from build123d import *

# Parameters (mm, degrees)
F0_R     = 9.525
F1_DEPTH = 6.35


with BuildPart() as f1:
    # F0 (on Front) → F1 (new body)
    with BuildSketch(Plane.XZ):
        with BuildLine():
            Line((0.076142, 15.237411), (0.853466, 15.24))
            Line((0.853466, 15.24), (45.610599, 15.24))
            ThreePointArc((45.610599, 15.24), (58.968483, 24.02141), (74.599698, 27.369742))
            ThreePointArc((74.599698, 27.369742), (81.067987, 24.723293), (84.296649, 18.525051))
            Line((84.296649, 18.525051), (140.869953, 18.525051))
            Line((140.869953, 18.525051), (140.869953, 1.794949))
            Line((140.869953, 1.794949), (140.869953, -1.794949))
            Line((140.869953, -1.794949), (140.869953, -18.525051))
            Line((140.869953, -18.525051), (84.296649, -18.525051))
            ThreePointArc((84.296649, -18.525051), (81.067987, -24.723293), (74.599698, -27.369742))
            ThreePointArc((74.599698, -27.369742), (58.968483, -24.02141), (45.610599, -15.24))
            Line((45.610599, -15.24), (0.853466, -15.24))
            Line((0.853466, -15.24), (0.076142, -15.237411))
            Line((0.076142, -15.237411), (0.000423, -37.973113))
            ThreePointArc((0.000423, -37.973113), (0.000106, -38.036556), (0, -38.1))
            ThreePointArc((0, -38.1), (5.576611, -51.567379), (19.041501, -57.149998))
            Line((19.041501, -57.149998), (107.941492, -57.189659))
            Line((107.941492, -57.189659), (148.581492, -46.300204))
            Line((148.581492, -46.300204), (164.745953, -30.135743))
            Line((164.745953, -30.135743), (164.745953, 1.837931))
            Line((164.745953, 1.837931), (164.745953, 30.135743))
            Line((164.745953, 30.135743), (148.581492, 46.300204))
            Line((148.581492, 46.300204), (107.941492, 57.189659))
            Line((107.941492, 57.189659), (51.653466, 57.164547))
            Line((51.653466, 57.164547), (19.041501, 57.149998))
            ThreePointArc((19.041501, 57.149998), (5.576611, 51.567379), (0, 38.1))
            ThreePointArc((0, 38.1), (0.000106, 38.036556), (0.000423, 37.973113))
            Line((0.000423, 37.973113), (0.076142, 15.237411))
        make_face()
        with Locations((19.05, -38.1)):
            Circle(F0_R, mode=Mode.SUBTRACT)
        with Locations((108.77014, -38.1)):
            Circle(F0_R, mode=Mode.SUBTRACT)
        with Locations((19.05, 38.1)):
            Circle(F0_R, mode=Mode.SUBTRACT)
        with Locations((108.77014, 38.1)):
            Circle(F0_R, mode=Mode.SUBTRACT)
        Polygon((51.653466, 57.189659), (51.653466, 57.164547), (107.941492, 57.189659), align=None)
    extrude(amount=F1_DEPTH)


solid = f1.part
Model file for the job. Use its own axes, mm. A direction names the side the tool comes from. Coordinates: 2 decimals unless noted, no trailing zeros. Write each loop counter-clockwise with the first axis right and the second up, starting at its lowest first coordinate (ties: lowest second). Pieces come first, ordered by that corner, then holes. Notation, with made-up numbers: (18.5, 28.5) -> (74.5, 28.5) arc R32 ccw to (74.5, 55.5) -> close; hole circle Ø3 at (-18, 22.25). An arc over 180 degrees is marked (long way). One line per item, written item: value. Start each with the question number.
1) Pull direction X, two halves, no side cores. Call faces 3 (the face through (24, -3, -15.24)), 4 (the face through (81.141, -3.131, -24.656)), 5 (the face through (5.43, -3.13, -51.42)): +X half, -X half, draft (parallel to the pull), parting line (faces both ways), or undercut.
2) Flat gauge pins, fed straight in: pin 1 Ø3 at (x, y) = (27.5, -2) entering from -Z; pin 2 Ø3 at (y, z) = (-3, -1.5) entering from -X; pin 3 Ø22 at (x, z) = (19.05, -38.1) entering from -Y; pin 4 Ø3 at (x, y) = (113, -4) entering from +Z. Where does each tip first touch, or does it go through?
3) Slice it at B-B on x = 69. Write the cut outline in (y, z), then the cut area to 3 significant figures.
4) Which spindle directions (+Z, -Z, +X, -X, +Y, -Y) get a long thin tool onto all of the face, cutting with end or side? Do faces 1 (the face through (59.18, -3.13, -24.11)), 2 (the face through (5.725, -3.131, 51.715)). Say none if no direction does.
5) Slice it at A-A on y = -1. Count the separate pieces of the cut face and the enclosed holes in it, then the cut area to 3 significant figures.
6) Slice it at C-C on z = -42. Write the cut outline in (x, y).
7) Probe probe 1 along Z at (x, y) = (19.05, -1.25) (3 decimals); probe 2 along Z at (x, y) = (19, -1.25); probe 3 along Z at (x, y) = (38, -1.25). List the from-to ranges inside material, lowest first.
8) Slice it at D-D on z = -21. Write the cut outline in (x, y), then the cut area to 3 significant figures.
Answers follow:
1. face 3: draft
1. face 4: undercut
1. face 5: -X half
2. pin 1: z = -57.15
2. pin 2: x = 140.87
2. pin 3: y = -6.35
2. pin 4: z = 56.24
3. outline: (-6.35, -57.17) -> (0, -57.17) -> (0, -26.86) -> (-6.35, -26.86) -> close; (-6.35, 26.86) -> (0, 26.86) -> (0, 57.19) -> (-6.35, 57.19) -> close
3. area: 385 mm2
4. face 1: +Y, -Y
4. face 2: +Z, -X, +Y, -Y
5. separate pieces: 1
5. enclosed holes: 4
5. area: 11,200 mm2
6. outline: (0.4, -6.35) -> (10.36, -6.35) -> (10.36, 0) -> (0.4, 0) -> close; (27.74, -6.35) -> (100.08, -6.35) -> (100.08, 0) -> (27.74, 0) -> close; (117.46, -6.35) -> (152.88, -6.35) -> (152.88, 0) -> (117.46, 0) -> close
7. probe 1: -57.15 to -47.625, -28.575 to -15.24, 15.24 to 28.575, 47.625 to 57.15
7. probe 2: -57.15 to -47.62, -28.58 to -15.24, 15.24 to 28.58, 47.62 to 57.15
7. probe 3: -57.16 to -15.24, 15.24 to 57.16
8. outline: (0.06, -6.35) -> (53.06, -6.35) -> (53.06, 0) -> (0.06, 0) -> close; (83.65, -6.35) -> (164.75, -6.35) -> (164.75, 0) -> (83.65, 0) -> close
8. area: 852 mm2
